Design review of the part built by this model. Coordinates are the model's own, in mm. Face numbers are marked on the shaded views. Round coordinates to 2 decimals unless told otherwise and drop trailing zeros. Order: outer loops, then holes, each group sorted by start corner. A loop starts at its lowest first (then second) coordinate and runs counter-clockwise, first axis right, second up.
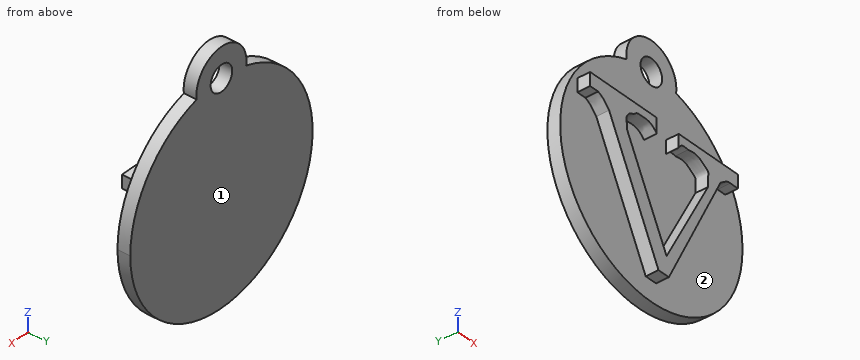
from build123d import *

# Parameters (mm, degrees)
F2_DEPTH = 4
F3_DEPTH = 8
F4_D     = 8


with BuildPart() as f2:
    # F0 (on Front) → F2 (new body)
    with BuildSketch(Plane.XZ):
        with BuildLine():
            ThreePointArc((-14.5860280627, 37.3082353296), (-25.7721388072, -22.1079707805), (28.3610324481, 4.8181205057))
            ThreePointArc((28.3610324481, 4.8181205057), (21.5239565547, 25.1881245814), (3.7817585998, 37.3082353296))
            ThreePointArc((3.7817585998, 37.3082353296), (-5.4021347314, 38.5812876852), (-14.5860280627, 37.3082353296))
        make_face()
        with BuildLine():
            ThreePointArc((-14.5860280627, 37.3082353296), (-5.4021347314, 38.5812876852), (3.7817585998, 37.3082353296))
            ThreePointArc((3.7817585998, 37.3082353296), (-5.4021347314, 47.8529951342), (-14.5860280627, 37.3082353296))
        make_face()
    extrude(amount=F2_DEPTH)

    # F1 (on Front) → F3 (join)
    with BuildSketch(Plane.XZ):
        with BuildLine():
            Line((-4.4812308624, -16.8456733227), (-19.2153304815, 12.5339938145))
            add(Edge.make_bspline(
                [(-19.2153304815, 12.5339938145), (-19.187462489, 13.0831996069), (-19.1294936303, 14.2256153377), (-19.5971693345, 16.2617964648), (-17.8782485083, 17.9666592712), (-16.6275418026, 18.0902554056), (-15.6181704414, 19.3512209953), (-13.9181197744, 19.2424127885), (-11.7824548248, 19.4327511912), (-9.7234432074, 18.78281747), (-8.6760339336, 17.6903028041), (-8.1412922591, 17.1325331371)],
                knots=[0, 0, 0, 0, 0.1071084643, 0.2227988055, 0.3430054249, 0.4340300552, 0.531806279, 0.6362553536, 0.7573294755, 0.8761076058, 1, 1, 1, 1], degree=3))
            Line((-8.1412922591, 17.1325331371), (-8.1412922591, 21.8196045607))
            Line((-8.1412922591, 21.8196045607), (-32.823253423, 21.8196045607))
            Line((-32.823253423, 21.8196045607), (-32.823253423, 17.6903028041))
            Line((-32.823253423, 17.6903028041), (-29.82012555, 17.6903028041))
            add(Edge.make_bspline(
                [(-29.82012555, 17.6903028041), (-29.2063598721, 17.3976096984), (-28.0591181767, 16.8505120895), (-27.1198992634, 15.6946853483), (-26.2472646135, 14.852226462), (-25.7846731693, 14.4056314602)],
                knots=[0, 0, 0, 0, 0.3509068735, 0.6559099195, 1, 1, 1, 1], degree=3))
            Line((-25.7846731693, 14.4056314602), (-7.4853163581, -22.570386529))
            Line((-7.4853163581, -22.570386529), (-3.6366009153, -22.570386529))
            Line((-3.6366009153, -22.570386529), (15.5083434656, 15.6256519258))
            add(Edge.make_bspline(
                [(15.5083434656, 15.6256519258), (16.0368847546, 16.0146436885), (17.0238298067, 16.7410079357), (18.3620600475, 17.5065309977), (18.870715753, 17.4367319386), (19.0745573491, 17.4087602645)],
                knots=[0, 0, 0, 0, 0.4086138264, 0.763004523, 1, 1, 1, 1], degree=3))
            Line((19.0745573491, 17.4087602645), (21.9529736787, 17.4087602645))
            Line((21.9529736787, 17.4087602645), (21.9529736787, 21.5079374611))
            Line((21.9529736787, 21.5079374611), (0, 21.5079374611))
            Line((0, 21.5079374611), (0, 17.4087602645))
            add(Edge.make_bspline(
                [(0, 17.4087602645), (0.3386937554, 17.949393323), (1.0610240671, 19.1023984773), (2.6512466921, 18.8543631276), (3.4958291799, 18.7226291746)],
                knots=[0, 0, 0, 0, 0.4688904091, 1, 1, 1, 1], degree=3))
            add(Edge.make_bspline(
                [(10.9098004177, 11.8717420846), (10.9188597305, 12.4813561639), (10.935968454, 13.6326265761), (10.8225562165, 15.0366139564), (11.2426073131, 16.3445815867), (9.2157140004, 17.5146925888), (7.9119458784, 18.5112803322), (6.2229710967, 18.9887989549), (4.9082762613, 18.9351899547), (3.9727099672, 18.7943955108), (3.4958291799, 18.7226291746)],
                knots=[0, 0, 0, 0, 0.1338160834, 0.2527147957, 0.3590610282, 0.503128831, 0.6364791552, 0.7657092985, 0.880576358, 1, 1, 1, 1], degree=3))
            Line((10.9098004177, 11.8717420846), (-4.4812308624, -16.8456733227))
        make_face()
    extrude(amount=F3_DEPTH)

    # F4 (through all)
    with Locations(Plane(origin=(0, 0, 0), x_dir=(1, 0, 0), z_dir=(0, 1, 0))):
        with Locations((-5.4021347314, -38.5812876852)):
            Hole(F4_D / 2)


solid = f2.part
1) The part is to be moulded in two halves that separate along X. For the marked faces 1 and 2, say which applies: released by +X, released by -X, zero draft, split by the parting line, or undercut.
Results:
face 1: zero draft
face 2: undercut
2) Take a section at C-C on z = 8. Give the boundary of the cut face in (x, y).
Results:
outline: (-39.02, -4) - (-22.61, -4) - (-22.61, -8) - (-16.94, -8) - (-16.94, -4) - (8.83, -4) - (8.83, -8) - (11.69, -8) - (11.69, -4) - (28.21, -4) - (28.21, 0) - (-39.02, 0) - close
3) Take a section at B-B on z = -18. Give the boundary of the cut face in (x, y), plus the area to 3 significant figures.
Results:
outline: (-30.29, -4) - (-9.75, -4) - (-9.75, -8) - (-1.35, -8) - (-1.35, -4) - (19.48, -4) - (19.48, 0) - (-30.29, 0) - close
area: 233 mm2
4) Take a section at A-A on x = -5.5. Give the boundary of the cut face in (y, z), plus the area to 3 significant figures.
Results:
outline: (-8, -22.57) - (-4, -22.57) - (-4, -28.94) - (0, -28.94) - (0, 34.58) - (-4, 34.58) - (-4, -14.81) - (-8, -14.81) - close; (-4, 42.58) - (0, 42.58) - (0, 47.85) - (-4, 47.85) - close
area: 306 mm2
5) To check wall thickness, follow line 1 along Y through (x, z) = (-14.5, 15); line 2 along Z through (x, y) = (-14, -6.5); line 3 along Z through (x, y) = (3, -4.75). State the ranges of each line that lie inside material, in increasing order.
Results:
line 1: y = -4 to 0
line 2: z = -9.41 to 2.13, 19.29 to 21.82
line 3: z = -9.33 to -2.89, 18.8 to 21.51
6) Take a section at D-D on z = 31. Give the boundary of the cut face in (x, y).
Results:
outline: (-26.72, -4) - (15.92, -4) - (15.92, 0) - (-26.72, 0) - close
7) Clearance check with flat-ended pins moving along their axes: P1, Ø4.5, axis at x = 15, y = -6.5, coming from the +Z side; P2, Ø1.2, axis at x = -18, y = -6, coming from the +Z side; P3, Ø1.4, axis at x = 20.5, y = -5.5, coming from the -Z side. State where each tip first meets the part, or that it passes through.
Results:
P1: stops at z = 21.51
P2: stops at z = 21.82
P3: stops at z = 17.41
